Check sheet for the modelled part. Datum: model origin and axes. Units: mm. A direction names the side the tool comes from. Round coordinates to 2 decimals unless told otherwise and drop trailing zeros. Order: outer loops, then holes, each group sorted by start corner. A loop starts at its lowest first (then second) coordinate and runs counter-clockwise, first axis right, second up. Notation, with made-up numbers: (-21, 18) -> (32, 18) arc R29 ccw to (32, 55) -> close; hole circle Ø8 at (62, 48.25). An arc over 180 degrees is marked (long way). Use CSV: the item, a comma, the result in double quotes.
```python
from build123d import *

# Parameters (mm, degrees)
SKETCH1_W                = 7.9
SKETCH1_H                = 95.7
BOSS_EXTRUDE1_DEPTH      = 9.2
SKETCH1_3_W              = 7.9
SKETCH1_3_H              = 95.7
BOSS_EXTRUDE2_DEPTH      = 9.2
BOSS_EXTRUDE3_DEPTH      = 32
BOSS_EXTRUDE3_DEPTH_BACK = 16
SKETCH2_R                = 3.8


with BuildPart() as part:
    # Sketch1 → Boss-Extrude1 (new body)
    with BuildSketch(Plane(origin=(0, 0, 0), x_dir=(0, 0, -1), z_dir=(1, 0, 0))):
        with Locations((-28.171698113, -0.670754717)):
            Rectangle(SKETCH1_W, SKETCH1_H)
    extrude(amount=BOSS_EXTRUDE1_DEPTH)

    # Sketch1_3 → Boss-Extrude2 (add)
    with BuildSketch(Plane(origin=(0, 0, 0), x_dir=(0, 0, -1), z_dir=(1, 0, 0))):
        with Locations((-28.171698113, -0.670754717)):
            Rectangle(SKETCH1_3_W, SKETCH1_3_H)
        with Locations((-4.071698113, -0.670754717)):
            Rectangle(SKETCH1_3_W, SKETCH1_3_H)
    extrude(amount=BOSS_EXTRUDE2_DEPTH)


with BuildPart() as boss_extrude2_piece_1:
    # of the separate pieces the step leaves, piece 1, a body of its own (boss_extrude2_pieces)
    add(part.part.solids().sort_by_distance((0, 47.179245283, 8.021698113))[0])



with BuildPart() as boss_extrude2_piece_2:
    # of the separate pieces the step leaves, piece 2, a body of its own (boss_extrude2_pieces)
    add(part.part.solids().sort_by_distance((0, 47.179245283, 32.121698113))[0])


with BuildPart() as boss_extrude2_piece_1_1:
    add(boss_extrude2_piece_1.part)

    add(boss_extrude2_piece_2.part)  # Boss-Extrude3 merges Boss-Extrude2 piece 2
    # Sketch2 → Boss-Extrude3 (add, two sides: drawn at the far end of the back side and taken through both)
    with BuildSketch(Plane.XY.offset(8.021698113).offset(-BOSS_EXTRUDE3_DEPTH_BACK)):
        with Locations(Location((4.3, 30.179245283, 0), (0, 0, 90))):
            Circle(SKETCH2_R)
    extrude(amount=BOSS_EXTRUDE3_DEPTH + BOSS_EXTRUDE3_DEPTH_BACK)


solid = boss_extrude2_piece_1_1.part
```
Q1. Sectioned sample at A-A, the plane y = 9. Enter the section's corners in (x, z), then the cut area to 3 significant figures.
Result sheet:
outline,"(0, 0.12) -> (9.2, 0.12) -> (9.2, 8.02) -> (0, 8.02) -> close; (0, 24.22) -> (9.2, 24.22) -> (9.2, 32.12) -> (0, 32.12) -> close"
area,"145 mm^2"
Q2. Sectioned sample at B-B, the plane x = 4.3. Enter the section's corners in (y, z), then the cut area to 3 significant figures.
Result sheet:
outline,"(-48.52, 0.12) -> (26.38, 0.12) -> (26.38, -7.98) -> (33.98, -7.98) -> (33.98, 0.12) -> (47.18, 0.12) -> (47.18, 8.02) -> (33.98, 8.02) -> (33.98, 24.22) -> (47.18, 24.22) -> (47.18, 32.12) -> (33.98, 32.12) -> (33.98, 40.02) -> (26.38, 40.02) -> (26.38, 32.12) -> (-48.52, 32.12) -> (-48.52, 24.22) -> (26.38, 24.22) -> (26.38, 8.02) -> (-48.52, 8.02) -> close"
area,"1,760 mm^2"
Q3. Access from +Z, -Z, +X, -X, +Y, -Y to the whole of each face (thin tool, end or side, straight path). Record for faces 1 (the face through (4.133, 26.383, 36.016)), 2 (the face through (4.133, 26.383, 16.008)), 3 (the face through (4.133, 26.383, -3.985)).
Result sheet:
face 1,"+Z"
face 2,"none"
face 3,"-Z"
Q4. Mould release check, pull along Z, two halves, no side actions. Record for faces 4 (the face through (4, 30, 40.022)), 5 (the face through (5, -1, 24.222)), 6 (the face through (9.2, 0, 28)), 7 (the face through (5, -1, 8.022)): pulls with the +Z half, pulls with the -Z half, needs draft (parallel to the pull), parting line crosses it, or undercut.
Result sheet:
face 4,"pulls with the +Z half"
face 5,"undercut"
face 6,"needs draft"
face 7,"undercut"
Q5. Sectioned sample at C-C, the plane y = 32.5. Enter the section's corners in (x, z), then the cut area to 3 significant figures.
Result sheet:
outline,"(0, 0.12) -> (1.29, 0.12) -> (1.29, -7.98) -> (7.31, -7.98) -> (7.31, 0.12) -> (9.2, 0.12) -> (9.2, 8.02) -> (7.31, 8.02) -> (7.31, 24.22) -> (9.2, 24.22) -> (9.2, 32.12) -> (7.31, 32.12) -> (7.31, 40.02) -> (1.29, 40.02) -> (1.29, 32.12) -> (0, 32.12) -> (0, 24.22) -> (1.29, 24.22) -> (1.29, 8.02) -> (0, 8.02) -> close"
area,"339 mm^2"
Q6. Go/stop test with flat-tipped pins: pin 1 (3 mm diameter, centred on x = 3, z = 23, fed in from +Y); pin 2 (4.5 mm diameter, centred on x = 3.5, y = 3, fed in from +Z). Record where each tip stops, or that it passes through.
Result sheet:
pin 1,"stops at y = 47.18"
pin 2,"stops at z = 32.12"
Q7. Scan lines: L1, parallel to Z at x = 6.25, y = 11.5; L2, parallel to Y at x = 4, z = 15; L3, parallel to Y at x = 2.5, z = 34. Record each from-to range of solid material in increasing order.
Result sheet:
L1,"z = 0.12 to 8.02, 24.22 to 32.12"
L2,"y = 26.39 to 33.97"
L3,"y = 26.83 to 33.53"
Q8. Sectioned sample at D-D, the plane z = 19.5. Enter the section's corners in (x, y).
Result sheet:
outline,"circle Ø7.6 at (4.3, 30.18)"
